Read the model definition and answer for the solid it produces. Units are mm, in the model's axes. A direction names the side the tool comes from. Round coordinates to 2 decimals unless told otherwise and drop trailing zeros. Loops run counter-clockwise (first coordinate to the right, second up) from the corner with the lowest first, then second, coordinate; pieces in that order, holes last. Notation, with made-up numbers: (18, 46) - (52, 46) arc R17 ccw to (52, 71) - close; hole circle Ø6 at (44.5, -19.75). An arc over 180 degrees is marked (long way). Use CSV: the item, a comma, the result in double quotes. Start each with the question number.
1. Consider line 1 along Y through (x, z) = (21, 59); line 2 along X through (y, z) = (-21, -46); line 3 along Z through (x, y) = (41.5, -17.5). Determine where each line is inside the solid, lowest interval first.
2. A tool of negligible diameter and unlimited length cuts with its end or side. For faces 4 (the cylindrical face through (-64.125, -15.776, 21.935)), 5 (the cylindrical face through (24.18, -16.79, -58.96)), 6 (the cylindrical face through (41, -17, -48)), 7 (the cylindrical face through (61.814, -16.79, -14.744)), from which of +Z, -Z, +X, -X, +Y, -Y can it reach the whole face along a straight path? Write none if from no direction.
3. Find section D-D (z = 35). Give the vertices of the cut face in (x, y), and give its area (3 significant figures).
4. Given pin 1 Ø8 at (x, y) = (-24.5, -10.5) entering from -Z; pin 2 Ø6 at (x, y) = (-7, -12.5) entering from +Z; pin 3 Ø6 at (y, z) = (-10.5, 43.5) entering from -X, each flat-ended and moving along its own axis, determine where each tip first touches the part or whether it passes through.
5. Find section B-B (y = -13). State how many separate pieces and enclosed holes the cut face has, and give its area (3 significant figures).
6. Find section C-C (x = 8.5). Give the vertices of the cut face in (y, z), and give its area (3 significant figures).
7. Find section A-A (z = 0). Give the vertices of the cut face in (x, y).
8. Determine the mould class of faces 1 (the cylindrical face through (-48.6, -16.79, -41.217)), 2 (the cylindrical face through (48.6, -16.79, 41.217)), 3 (the cylindrical face through (27.5, -15.78, -58.41)) for opening direction X: +X half, -X half, draft (parallel to the pull), parting line (faces both ways), or undercut.
from build123d import *
from build123d.topology import SkipClean

# Parameters (mm, degrees)
SKETCH1_R           = 70
BOSS_EXTRUDE1_DEPTH = 2
SKETCH2_R           = 7.525
CUT_EXTRUDE1_DEPTH  = 2
SKETCH3_R           = 7.525
BOSS_EXTRUDE3_DEPTH = 32
SKETCH4_R           = 70
BOSS_EXTRUDE4_DEPTH = 2


with BuildPart() as part:
    # Sketch1 → Boss-Extrude1 (new body)
    with BuildSketch(Plane(origin=(0, 0, 0), x_dir=(1, 0, 0), z_dir=(0, 1, 0))):
        with Locations(Location((0, 0, 0), (0, 0, 270))):
            Circle(SKETCH1_R)
    extrude(amount=-BOSS_EXTRUDE1_DEPTH)

    # Sketch2 → Cut-Extrude1 (cut)
    with BuildSketch(Plane(origin=(0, 0, 0), x_dir=(1, 0, 0), z_dir=(0, 1, 0))):
        with Locations(Location((-56.77852978, -23.566378191, 0), (0, 0, 270))):
            Circle(SKETCH2_R)
        with Locations(Location((-59.786765058, 14.307982, 0), (0, 0, 270))):
            Circle(SKETCH2_R)
        with Locations(Location((-39.958488161, 46.717179376, 0), (0, 0, 270))):
            Circle(SKETCH2_R)
        with Locations(Location((-4.867426926, 61.28200209, 0), (0, 0, 270))):
            Circle(SKETCH2_R)
        with Locations(Location((32.082825957, 52.439182904, 0), (0, 0, 270))):
            Circle(SKETCH2_R)
        with Locations(Location((56.77852978, 23.566378191, 0), (0, 0, 270))):
            Circle(SKETCH2_R)
        with Locations(Location((59.786765058, -14.307982, 0), (0, 0, 270))):
            Circle(SKETCH2_R)
        with Locations(Location((39.958488161, -46.717179376, 0), (0, 0, 270))):
            Circle(SKETCH2_R)
        with Locations(Location((4.867426926, -61.28200209, 0), (0, 0, 270))):
            Circle(SKETCH2_R)
        with Locations(Location((-32.082825957, -52.439182904, 0), (0, 0, 270))):
            Circle(SKETCH2_R)
    extrude(amount=-CUT_EXTRUDE1_DEPTH, mode=Mode.SUBTRACT)

    # Sketch3 → Boss-Extrude3 (add)
    # profile 1 of 10: a face of its own
    with BuildSketch(Plane(origin=(0, 0, 0), x_dir=(1, 0, 0), z_dir=(0, 1, 0))):
        with BuildLine():
            ThreePointArc((-53.839060138, 44.73651309), (-48.521333413, 41.173599259), (-42.648435641, 38.627691904))
            ThreePointArc((-42.648435641, 38.627691904), (-42.620662511, 38.618509564), (-42.592858038, 38.609422575))
            ThreePointArc((-42.592858038, 38.609422575), (-34.417274472, 40.238709198), (-31.540375481, 48.06291483))
            ThreePointArc((-31.540375481, 48.06291483), (-31.545042632, 48.091791807), (-31.549808841, 48.120652599))
            ThreePointArc((-31.549808841, 48.120652599), (-33.15457894, 54.317206918), (-35.850120348, 60.122947957))
            ThreePointArc((-35.850120348, 60.122947957), (-45.499701851, 53.195649554), (-53.839060138, 44.73651309))
        make_face()
        with Locations(Location((-39.958488161, 46.717179376, 0), (0, 0, 270))):
            Circle(SKETCH3_R, mode=Mode.SUBTRACT)
    # profile 2 of 10: a face of its own
    with BuildSketch(Plane(origin=(0, 0, 0), x_dir=(1, 0, 0), z_dir=(0, 1, 0))):
        with BuildLine():
            ThreePointArc((-53.80894145, 20.385913384), (-58.749470976, 24.455770937), (-64.342738745, 27.568314616))
            ThreePointArc((-64.342738745, 27.568314616), (-68.07765033, 16.292130784), (-69.852177246, 4.546793813))
            ThreePointArc((-69.852177246, 4.546793813), (-63.455817749, 4.790017318), (-57.208096848, 6.182337701))
            ThreePointArc((-57.208096848, 6.182337701), (-57.18023067, 6.191233667), (-57.152395181, 6.200225198))
            ThreePointArc((-57.152395181, 6.200225198), (-51.495879786, 12.323833215), (-53.767372292, 20.344747337))
            ThreePointArc((-53.767372292, 20.344747337), (-53.788121558, 20.365366019), (-53.80894145, 20.385913384))
        make_face()
        with Locations(Location((-59.786765058, 14.307982, 0), (0, 0, 270))):
            Circle(SKETCH3_R, mode=Mode.SUBTRACT)
    # profile 3 of 10: a face of its own
    with BuildSketch(Plane(origin=(0, 0, 0), x_dir=(1, 0, 0), z_dir=(0, 1, 0))):
        with BuildLine():
            ThreePointArc((-55.514887324, -15.135551852), (-61.90406192, -14.746938322), (-68.258617871, -15.516477896))
            ThreePointArc((-68.258617871, -15.516477896), (-64.652250258, -26.834428196), (-59.184136835, -37.379646161))
            ThreePointArc((-59.184136835, -37.379646161), (-54.152336488, -33.423188431), (-49.916209492, -28.624459374))
            ThreePointArc((-49.916209492, -28.624459374), (-49.898894198, -28.600883058), (-49.881659903, -28.577247466))
            ThreePointArc((-49.881659903, -28.577247466), (-48.904809302, -20.298328185), (-55.457060374, -15.144422147))
            ThreePointArc((-55.457060374, -15.144422147), (-55.48596624, -15.139937394), (-55.514887324, -15.135551852))
        make_face()
        with Locations(Location((-56.77852978, -23.566378191, 0), (0, 0, 270))):
            Circle(SKETCH3_R, mode=Mode.SUBTRACT)
    # profile 4 of 10: a face of its own
    with BuildSketch(Plane(origin=(0, 0, 0), x_dir=(1, 0, 0), z_dir=(0, 1, 0))):
        with BuildLine():
            ThreePointArc((-36.016033123, -44.87575072), (-41.413405253, -48.316818371), (-46.102024996, -52.674503237))
            ThreePointArc((-46.102024996, -52.674503237), (-36.531888036, -59.711147674), (-25.909767747, -65.028331789))
            ThreePointArc((-25.909767747, -65.028331789), (-24.16450326, -58.869872212), (-23.558026699, -52.497685878))
            ThreePointArc((-23.558026699, -52.497685878), (-23.557876143, -52.468434563), (-23.557825957, -52.439182904))
            ThreePointArc((-23.557825957, -52.439182904), (-27.633763879, -45.167218133), (-35.964036308, -44.84893711))
            ThreePointArc((-35.964036308, -44.84893711), (-35.990057717, -44.862299311), (-36.016033123, -44.87575072))
        make_face()
        with Locations(Location((-32.082825957, -52.439182904, 0), (0, 0, 270))):
            Circle(SKETCH3_R, mode=Mode.SUBTRACT)
    # profile 5 of 10: a face of its own
    with BuildSketch(Plane(origin=(0, 0, 0), x_dir=(1, 0, 0), z_dir=(0, 1, 0))):
        with BuildLine():
            ThreePointArc((-2.760278408, -57.474938084), (-5.104235368, -63.431316031), (-6.336025522, -69.712658683))
            ThreePointArc((-6.336025522, -69.712658683), (5.542413742, -69.780238248), (17.261251979, -67.838404905))
            ThreePointArc((17.261251979, -67.838404905), (15.053348893, -61.830265722), (11.798521586, -56.318580708))
            ThreePointArc((11.798521586, -56.318580708), (11.781449896, -56.294827402), (11.764296803, -56.271132814))
            ThreePointArc((11.764296803, -56.271132814), (4.192440109, -52.783765932), (-2.733972746, -57.422682456))
            ThreePointArc((-2.733972746, -57.422682456), (-2.747170403, -57.448787704), (-2.760278408, -57.474938084))
        make_face()
        with Locations(Location((4.867426926, -61.28200209, 0), (0, 0, 270))):
            Circle(SKETCH3_R, mode=Mode.SUBTRACT)
    # profile 6 of 10: a face of its own
    with BuildSketch(Plane(origin=(0, 0, 0), x_dir=(1, 0, 0), z_dir=(0, 1, 0))):
        with BuildLine():
            ThreePointArc((31.549808841, -48.1206526), (33.15457894, -54.317206918), (35.850120348, -60.122947957))
            ThreePointArc((35.850120348, -60.122947957), (45.499701851, -53.195649554), (53.839060138, -44.73651309))
            ThreePointArc((53.839060138, -44.73651309), (48.521333413, -41.173599259), (42.648435641, -38.627691905))
            ThreePointArc((42.648435641, -38.627691905), (42.620662512, -38.618509564), (42.592858038, -38.609422575))
            ThreePointArc((42.592858038, -38.609422575), (34.417274472, -40.238709198), (31.540375481, -48.06291483))
            ThreePointArc((31.540375481, -48.06291483), (31.545042633, -48.091791807), (31.549808841, -48.1206526))
        make_face()
        with Locations(Location((39.958488161, -46.717179376, 0), (0, 0, 270))):
            Circle(SKETCH3_R, mode=Mode.SUBTRACT)
    # profile 7 of 10: a face of its own
    with BuildSketch(Plane(origin=(0, 0, 0), x_dir=(1, 0, 0), z_dir=(0, 1, 0))):
        with BuildLine():
            ThreePointArc((64.342738745, -27.568314616), (68.07765033, -16.292130784), (69.852177246, -4.546793813))
            ThreePointArc((69.852177246, -4.546793813), (63.455817749, -4.790017318), (57.208096849, -6.182337701))
            ThreePointArc((57.208096849, -6.182337701), (57.180230671, -6.191233667), (57.152395181, -6.200225198))
            ThreePointArc((57.152395181, -6.200225198), (51.495879786, -12.323833215), (53.767372292, -20.344747337))
            ThreePointArc((53.767372292, -20.344747337), (53.788121559, -20.36536602), (53.808941451, -20.385913385))
            ThreePointArc((53.808941451, -20.385913385), (58.749470976, -24.455770937), (64.342738745, -27.568314616))
        make_face()
        with Locations(Location((59.786765058, -14.307982, 0), (0, 0, 270))):
            Circle(SKETCH3_R, mode=Mode.SUBTRACT)
    # profile 8 of 10: a face of its own
    with BuildSketch(Plane(origin=(0, 0, 0), x_dir=(1, 0, 0), z_dir=(0, 1, 0))):
        with BuildLine():
            ThreePointArc((68.258617871, 15.516477896), (64.652250258, 26.834428196), (59.184136835, 37.379646161))
            ThreePointArc((59.184136835, 37.379646161), (54.152336489, 33.423188431), (49.916209492, 28.624459375))
            ThreePointArc((49.916209492, 28.624459375), (49.898894198, 28.600883058), (49.881659903, 28.577247466))
            ThreePointArc((49.881659903, 28.577247466), (48.904809302, 20.298328185), (55.457060374, 15.144422147))
            ThreePointArc((55.457060374, 15.144422147), (55.48596624, 15.139937394), (55.514887325, 15.135551852))
            ThreePointArc((55.514887325, 15.135551852), (61.904061921, 14.746938322), (68.258617871, 15.516477896))
        make_face()
        with Locations(Location((56.77852978, 23.566378191, 0), (0, 0, 270))):
            Circle(SKETCH3_R, mode=Mode.SUBTRACT)
    # profile 9 of 10: a face of its own
    with BuildSketch(Plane(origin=(0, 0, 0), x_dir=(1, 0, 0), z_dir=(0, 1, 0))):
        with BuildLine():
            ThreePointArc((46.102024996, 52.674503237), (36.531888036, 59.711147674), (25.909767747, 65.028331789))
            ThreePointArc((25.909767747, 65.028331789), (24.16450326, 58.869872212), (23.558026699, 52.497685879))
            ThreePointArc((23.558026699, 52.497685879), (23.557876143, 52.468434563), (23.557825957, 52.439182904))
            ThreePointArc((23.557825957, 52.439182904), (27.633763879, 45.167218133), (35.964036308, 44.84893711))
            ThreePointArc((35.964036308, 44.84893711), (35.990057717, 44.862299311), (36.016033123, 44.87575072))
            ThreePointArc((36.016033123, 44.87575072), (41.413405253, 48.316818371), (46.102024996, 52.674503237))
        make_face()
        with Locations(Location((32.082825957, 52.439182904, 0), (0, 0, 270))):
            Circle(SKETCH3_R, mode=Mode.SUBTRACT)
    # profile 10 of 10: a face of its own
    with BuildSketch(Plane(origin=(0, 0, 0), x_dir=(1, 0, 0), z_dir=(0, 1, 0))):
        with BuildLine():
            ThreePointArc((6.336025522, 69.712658683), (-5.542413742, 69.780238248), (-17.261251979, 67.838404905))
            ThreePointArc((-17.261251979, 67.838404905), (-15.053348893, 61.830265721), (-11.798521586, 56.318580707))
            ThreePointArc((-11.798521586, 56.318580707), (-11.781449896, 56.294827402), (-11.764296803, 56.271132814))
            ThreePointArc((-11.764296803, 56.271132814), (-4.192440109, 52.783765932), (2.733972746, 57.422682456))
            ThreePointArc((2.733972746, 57.422682456), (2.747170402, 57.448787704), (2.760278407, 57.474938083))
            ThreePointArc((2.760278407, 57.474938083), (5.104235368, 63.431316031), (6.336025522, 69.712658683))
        make_face()
        with Locations(Location((-4.867426926, 61.28200209, 0), (0, 0, 270))):
            Circle(SKETCH3_R, mode=Mode.SUBTRACT)
    extrude(amount=-BOSS_EXTRUDE3_DEPTH)

    # Sketch4 → Boss-Extrude4 (add)
    with SkipClean():  # the faces are left unmerged after this step: merging them gives an invalid solid
        with BuildSketch(Plane.XZ.offset(32)):
            with Locations(Location((0, 0, 0), (0, 0, 90))):
                Circle(SKETCH4_R)
        extrude(amount=BOSS_EXTRUDE4_DEPTH)
    add(part.part.scale(1), mode=Mode.REPLACE)  # the faces are merged on a copy


solid = part.part
Filled sheet:
1,line 1,"y = -34 to -32, -2 to 0"
1,line 2,"x = -52.76 to -47.45, -32.47 to -31.46, 26.5 to 28.19, 35.98 to 38.03"
1,line 3,"z = -56.37 to -48.38, 38.33 to 39.35, 54.08 to 56.37"
2,face 4,"+Y"
2,face 5,"-Z"
2,face 6,"+X"
2,face 7,"none"
3,outline,"(-60.62, -34) - (60.62, -34) - (60.62, -32) - (-55.94, -32) - (-55.94, -2) - (60.62, -2) - (60.62, 0) - (-60.62, 0) - close"
3,area,"625 mm²"
4,pin 1,"stops at z = 44.7"
4,pin 2,"stops at z = 69.89"
4,pin 3,"stops at x = -38.83"
5,separate pieces,"10"
5,enclosed holes,"10"
5,area,"1,190 mm²"
6,outline,"(-34, -69.48) - (-32, -69.48) - (-32, 53.57) - (-2, 53.57) - (-2, -69.48) - (0, -69.48) - (0, 54.69) - (-32, 54.69) - (-32, 67.87) - (0, 67.87) - (0, 69.48) - (-34, 69.48) - close"
6,area,"611 mm²"
7,outline,"(-70, -34) - (70, -34) - (70, -32) - (-70, -32) - close; (-70, -2) - (70, -2) - (70, 0) - (-70, 0) - close"
8,face 1,"-X half"
8,face 2,"+X half"
8,face 3,"undercut"
